```python
from build123d import *

# Parameters (mm, degrees)
F0_W     = 59.436
F0_H     = 44.45
F0_W_2   = 7.62
F0_W_3   = 18.288
F1_DEPTH = 7.62
F2_DEPTH = 15.24
F3_F1_R  = 5.08
F3_F2_R  = 5.08


with BuildPart() as f1:
    # F0 (on Top) → F1 (new body)
    with BuildSketch(Plane.XY):
        with Locations((-46.482, 0)):
            Rectangle(F0_W, F0_H)
        with Locations((-12.954, 0)):
            Rectangle(F0_W_2, F0_H)
        Rectangle(F0_W_3, F0_H)
        with Locations((12.954, 0)):
            Rectangle(F0_W_2, F0_H)
        with Locations((46.482, 0)):
            Rectangle(F0_W, F0_H)
    extrude(amount=-F1_DEPTH)

    # F0 (on Top) → F2 (join)
    with BuildSketch(Plane.XY):
        with Locations((-12.954, 0)):
            Rectangle(F0_W_2, F0_H)
        with Locations((12.954, 0)):
            Rectangle(F0_W_2, F0_H)
    extrude(amount=F2_DEPTH)

    # F3: fillet of radius 5.08 on 8 edges, made by hand

    # F3_f1
    f3_f1_edges = [f1.edges().sort_by_distance(p)[0] for p in [
        (16.764, 0, 0),
        (-16.764, 0, 0),
    ]]
    fillet(f3_f1_edges, radius=F3_F1_R)

    # F3_f2
    f3_f2_edges = [f1.edges().sort_by_distance(p)[0] for p in [
        (49.022, 22.225, 0),
        (76.2, 0, 0),
        (49.022, -22.225, 0),
        (-49.022, 22.225, 0),
        (-49.022, -22.225, 0),
        (-76.2, 0, 0),
        (-18.2518975516, -22.225, 1.4878975516),
        (-18.2518975516, 22.225, 1.4878975516),
        (18.2518975516, -22.225, 1.4878975516),
        (18.2518975516, 22.225, 1.4878975516),
    ]]
    fillet(f3_f2_edges, radius=F3_F2_R)


solid = f1.part
```
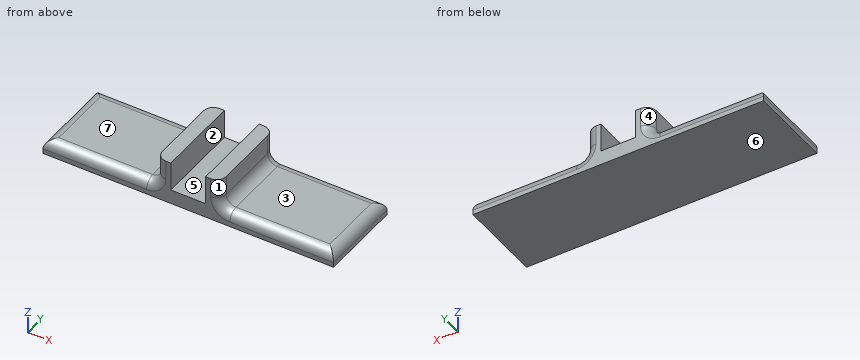
Design review of the part built by this model. Coordinates are the model's own, in mm. Face numbers are marked on the shaded views. A direction names the side the tool comes from. Give positions to 0.01 mm unless a question says otherwise; leave off trailing zeros. Loops run counter-clockwise (first coordinate to the right, second up) from the corner with the lowest first, then second, coordinate; pieces in that order, holes last. Notation, with made-up numbers: (-21, -29) -> (-2, -29) arc R4 cw to (-2, -22) -> close; hole circle Ø3 at (79, -17). An arc over 180 degrees is marked (long way). One line per item, written item: value.
Q1. For L1, parallel to X at y = -15, z = 13.5; L2, parallel to Z at x = 44, y = -1.5; L3, parallel to X at y = 2, z = -4.75, list the stretches that pass through material, from the lowest coordinate up.
Numbers:
L1: x = -16.76 to -9.14, 9.14 to 16.76
L2: z = -7.62 to 0
L3: x = -76.19 to 76.19
Q2. Machinability: for the marked faces 4, 5, 6 and 7, which of the approach directions +Z, -Z, +X, -X, +Y, -Y give a long, thin tool a straight path to every point of the face, cutting with its end or side? Answer none if there is none.
Numbers:
face 4: +Z, -X, +Y
face 5: +Z, +Y, -Y
face 6: -Z, +X, -X, +Y, -Y
face 7: +Z, -X, +Y, -Y
Q3. We need section B-B on y = 6.5. Give the boundary of the cut face in (x, z), and give its area (3 significant figures).
Numbers:
outline: (-76.2, -7.62) -> (76.2, -7.62) -> (76.2, -5.08) arc R5.08 ccw to (71.12, 0) -> (21.84, 0) arc R5.08 cw to (16.76, 5.08) -> (16.76, 15.24) -> (9.14, 15.24) -> (9.14, 0) -> (-9.14, 0) -> (-9.14, 15.24) -> (-16.76, 15.24) -> (-16.76, 5.08) arc R5.08 cw to (-21.84, 0) -> (-71.12, 0) arc R5.08 ccw to (-76.2, -5.08) -> close
area: 1,390 mm^2
Q4. Draft analysis for pull direction X (two halves, no side actions). For the marked faces 1, 2 and 3, state which applies: pulls with the +X half, pulls with the -X half, needs draft (parallel to the pull), parting line crosses it, or undercut.
Numbers:
face 1: pulls with the +X half
face 2: undercut
face 3: needs draft
Q5. We need section A-A on z = 12.5. Give the boundary of the cut face in (x, y) (3 decimals).
Numbers:
outline: (-16.764, -17.145) arc R5.08 ccw to (-11.684, -22.225) -> (-9.144, -22.225) -> (-9.144, 22.225) -> (-11.684, 22.225) arc R5.08 ccw to (-16.764, 17.145) -> close; (9.144, -22.225) -> (11.684, -22.225) arc R5.08 ccw to (16.764, -17.145) -> (16.764, 17.145) arc R5.08 ccw to (11.684, 22.225) -> (9.144, 22.225) -> close
Q6. For pin 1 Ø1.5 at (x, y) = (53.5, 14) entering from +Z; pin 2 Ø4 at (y, z) = (-16, 8.5) entering from -X; pin 3 Ø10 at (x, z) = (-60, 9.5) entering from +Y; pin 4 Ø4 at (x, z) = (39, -2.5) entering from -Y, all flat-tipped, find the tip position at first contact; note any pin that passes through.
Numbers:
pin 1: stops at z = 0
pin 2: stops at x = -16.76
pin 3: passes through
pin 4: stops at y = -22.19
Q7. We need section C-C on x = -54. Give the boundary of the cut face in (y, z) (3 decimals).
Numbers:
outline: (-22.225, -7.62) -> (22.225, -7.62) -> (22.225, -5.08) arc R5.08 ccw to (17.145, 0) -> (-17.145, 0) arc R5.08 ccw to (-22.225, -5.08) -> close
